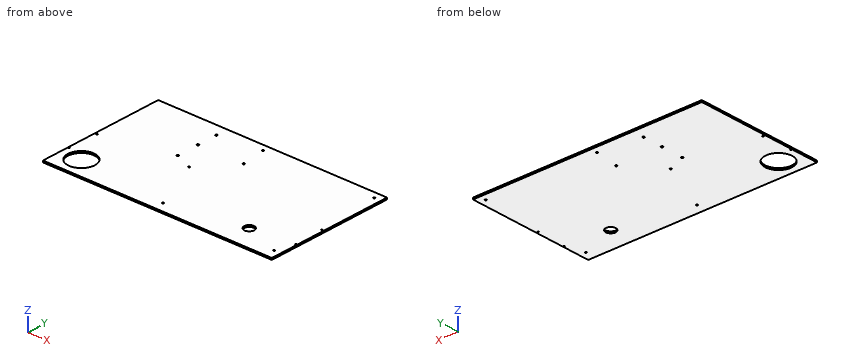
from build123d import *

# Parameters (mm, degrees)
SKETCH1_W           = 863.346
SKETCH1_H           = 482.219
SKETCH1_R           = 2.54
BOSS_EXTRUDE1_DEPTH = 6.35
SKETCH2_R           = 19.05
CUT_EXTRUDE1_DEPTH  = 495.485280286
SKETCH3_R           = 3.81
CUT_EXTRUDE2_DEPTH  = 495.485280286
SKETCH4_R           = 3.175
CUT_EXTRUDE3_DEPTH  = 495.485280286
SKETCH5_R           = 50.8
CUT_EXTRUDE4_DEPTH  = 495.485280286
SKETCH6_R           = 3.175
CUT_EXTRUDE5_DEPTH  = 495.485280286


with BuildPart() as part:
    # Sketch1 → Boss-Extrude1 (new body)
    with BuildSketch(Plane.XY):
        Rectangle(SKETCH1_W, SKETCH1_H)
        with Locations((-423.918892064, -23.561444512)):
            Circle(SKETCH1_R, mode=Mode.SUBTRACT)
        with Locations((-427.847603153, -135.890923479)):
            Circle(SKETCH1_R, mode=Mode.SUBTRACT)
        with Locations(Location((427.847603153, -135.890923479, 0), (0, 0, 180))):
            Circle(SKETCH1_R, mode=Mode.SUBTRACT)
        with Locations(Location((423.918892064, -23.561444512, 0), (0, 0, 180))):
            Circle(SKETCH1_R, mode=Mode.SUBTRACT)
    extrude(amount=BOSS_EXTRUDE1_DEPTH)

    # Sketch2 → Cut-Extrude1 (cut, through all)
    with BuildSketch(Plane.XY.offset(6.35)):
        with Locations((266.52855, -152.344105106)):
            Circle(SKETCH2_R)
    extrude(amount=-CUT_EXTRUDE1_DEPTH, mode=Mode.SUBTRACT)

    # Sketch3 → Cut-Extrude2 (cut, through all)
    with BuildSketch(Plane(origin=(0, 0, 0), x_dir=(-1, 0, 0), z_dir=(0, 0, -1))):
        with Locations((171.299738172, 195.628424293)):
            Circle(SKETCH3_R)
        with Locations((171.299738172, 118.638765896)):
            Circle(SKETCH3_R)
        with Locations((171.299738172, 33.532528438)):
            Circle(SKETCH3_R)
        with Locations((0.611738172, 121.072249047)):
            Circle(SKETCH3_R)
    extrude(amount=-CUT_EXTRUDE2_DEPTH, mode=Mode.SUBTRACT)

    # Sketch4 → Cut-Extrude3 (cut, through all)
    with BuildSketch(Plane.XY.offset(6.35)):
        with Locations((-12.827, 215.7095)):
            Circle(SKETCH4_R)
        with Locations((-12.827, -203.3905)):
            Circle(SKETCH4_R)
        with Locations((406.273, -203.3905)):
            Circle(SKETCH4_R)
        with Locations((406.273, 215.7095)):
            Circle(SKETCH4_R)
    extrude(amount=-CUT_EXTRUDE3_DEPTH, mode=Mode.SUBTRACT)

    # Sketch5 → Cut-Extrude4 (cut, through all)
    with BuildSketch(Plane.XY.offset(6.35)):
        with Locations((-355.473, -164.9095)):
            Circle(SKETCH5_R)
    extrude(amount=-CUT_EXTRUDE4_DEPTH, mode=Mode.SUBTRACT)

    # Sketch6 → Cut-Extrude5 (cut, through all)
    with BuildSketch(Plane.XY.offset(6.35)):
        with Locations((-101.473, 4.6355)):
            Circle(SKETCH6_R)
    extrude(amount=-CUT_EXTRUDE5_DEPTH, mode=Mode.SUBTRACT)


solid = part.part
Part model, mm, in its own coordinate system. Round coordinates to 2 decimals unless told otherwise and drop trailing zeros. Put each result on its own line as item: value.
Q1. Pin check, flat tips, straight feed: pin 1 Ø7.5 at (x, y) = (-12.83, 215.71) entering from -Z; pin 2 Ø4 at (x, y) = (-12.83, -203.39) entering from +Z. Stop position of each tip, or through.
From the geometry:
pin 1: stops at z = 0
pin 2: passes through
Q2. Wall check: line 1 (X direction, y = -143.5, z = 3.5); line 2 (X direction, y = 33, z = 4.75); line 3 (X direction, y = -177.5, z = 3.5). Give the ranges that are in metal, low to high. Write a range as [from, to].
From the geometry:
line 1: x = [-431.67, -401.54], [-309.4, 249.66], [283.4, 431.67]
line 2: x = [-431.67, -175.07], [-167.53, 431.67]
line 3: x = [-431.67, -404.69], [-306.26, 431.67]
Q3. Band-saw the part on A-A (z = 4.75). State how many separate pieces and enclosed holes the cut face has, and give its area (3 significant figures).
From the geometry:
separate pieces: 1
enclosed holes: 15
area: 407,000 mm2
